```python
from build123d import *

# Parameters (mm, degrees)
SKETCH1_R           = 2.35
BOSS_EXTRUDE1_DEPTH = 1.5
SKETCH2_R           = 1.25
BOSS_EXTRUDE2_DEPTH = 15
CHAMFER1_SIZE       = 1.1
CUT_EXTRUDE1_DEPTH  = 0.3


with BuildPart() as part:
    # Sketch1 → Boss-Extrude1 (new body)
    with BuildSketch(Plane(origin=(0, 0, 0), x_dir=(1, 0, 0), z_dir=(0, 1, 0))):
        with Locations(Location((0, 0, 0), (0, 0, 270))):
            Circle(SKETCH1_R)
    extrude(amount=BOSS_EXTRUDE1_DEPTH)

    # Sketch2 → Boss-Extrude2 (add)
    with BuildSketch(Plane.XZ):
        with Locations(Location((0, 0, 0), (0, 0, 270))):
            Circle(SKETCH2_R)
    extrude(amount=-BOSS_EXTRUDE2_DEPTH)

    # Chamfer1
    chamfer1_edges = [part.edges().sort_by_distance(p)[0] for p in [
        (0, 1.5, -2.35),
    ]]
    chamfer(chamfer1_edges, length=CHAMFER1_SIZE - 0.0001)  # a hair under: the kernel refuses the full size

    # Sketch3 → Cut-Extrude1 (cut)
    with BuildSketch(Plane.XZ):
        Polygon((-0.25, 1.5), (-0.25, 0.25), (-1.5, 0.25), (-1.5, -0.25), (-0.25, -0.25), (-0.25, -1.5), (0.25, -1.5), (0.25, -0.25), (1.5, -0.25), (1.5, 0.25), (0.25, 0.25), (0.25, 1.5), align=None)
    extrude(amount=-CUT_EXTRUDE1_DEPTH, mode=Mode.SUBTRACT)


solid = part.part
```
Can you work these out from the model? Positions are in its coordinate system, mm. Round coordinates to 2 decimals unless told otherwise and drop trailing zeros. Loops run counter-clockwise (first coordinate to the right, second up) from the corner with the lowest first, then second, coordinate; pieces in that order, holes last.
Item 1: Please list where these lines run through material, in increasing order: L1, parallel to X at y = 1.75, z = -0.1; L2, parallel to Y at x = -1.7, z = -0.05; L3, parallel to X at y = 11.75, z = -0.7.
Item 2: Will these pins go through, and if not, where does the flat tip stop? pin 1 Ø1.5 at (y, z) = (12, 0) entering from -X; pin 2 Ø1.5 at (x, y) = (1, 3) entering from +Z.
Item 3: Suppose I cut it at C-C, the plane y = 5.75. Write out the boundary of the cut face in (x, z), then the cut area to 3 significant figures.
Item 4: If we mould it in two halves opening along X, with no side actions, what happens to faces 1 (the flat face through (0, 0.3, 0)), 2 (the cylindrical face through (-1.22, 8.16, 0.27)), 3 (the flat face through (-0.5, 0, -0.5))? For each: +X half, -X half, draft (parallel to the pull), parting line (faces both ways), or undercut.
Reported:
1. L1: x = -1.25 to 1.25
1. L2: y = 0 to 1.05
1. L3: x = -1.04 to 1.04
2. pin 1: stops at x = -1.25
2. pin 2: stops at z = 1.22
3. outline: circle Ø2.5 at (0, 0)
3. area: 4.91 mm2
4. face 1: undercut
4. face 2: parting line
4. face 3: draft
